```python
from build123d import *

# Parameters (mm, degrees)
F0_R     = 6.35
F0_R_2   = 3.175
F1_DEPTH = 2.3749
F2_R     = 0.2032
F3_R     = 0.2032
F4_R     = 0.2032
F5_R     = 0.2032


with BuildPart() as f1:
    # F0 (on Right) → F1 (new body, symmetric)
    with BuildSketch(Plane.YZ):
        Circle(F0_R)
        Circle(F0_R_2, mode=Mode.SUBTRACT)
    extrude(amount=F1_DEPTH, both=True)

    # F2
    f2_edges = [f1.edges().sort_by_distance(p)[0] for p in [
        (2.3749, -6.35, 0),
    ]]
    fillet(f2_edges, radius=F2_R)

    # F3
    f3_edges = [f1.edges().sort_by_distance(p)[0] for p in [
        (2.3749, -3.175, 0),
    ]]
    fillet(f3_edges, radius=F3_R)

    # F4
    f4_edges = [f1.edges().sort_by_distance(p)[0] for p in [
        (-2.3749, -6.35, 0),
    ]]
    fillet(f4_edges, radius=F4_R)

    # F5
    f5_edges = [f1.edges().sort_by_distance(p)[0] for p in [
        (-2.3749, -3.175, 0),
    ]]
    fillet(f5_edges, radius=F5_R)


solid = f1.part
```
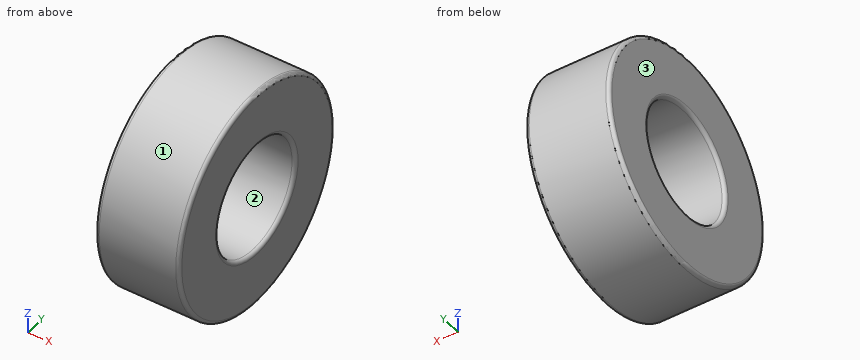
Part model, mm, in its own coordinate system. Face numbers are marked on the shaded views. Give positions to 0.01 mm unless a question says otherwise; leave off trailing zeros. Order: outer loops, then holes, each group sorted by start corner. A loop starts at its lowest first (then second) coordinate and runs counter-clockwise, first axis right, second up. Notation, with made-up numbers: (31, 44.5) - (55, 44.5) arc R30 ccw to (55, 68.5) - close; hole circle Ø4 at (15, 69.25). An arc over 180 degrees is marked (long way). Use one line per item in the form item = value.
Item 1: Slice it at C-C on x = 1.9. Give the cut face in (y, z) (3 decimals), and give its area (3 significant figures).
Solution:
outline = circle Ø12.7 at (0, 0); hole circle Ø6.35 at (0, 0)
area = 95.0 mm2
Item 2: Two-plate mould, pull along Z, no slides. Class the marked faces 1, 2 and 3: released by +Z, released by -Z, zero draft, split by the parting line, or undercut.
Solution:
face_1 = split by the parting line
face_2 = undercut
face_3 = zero draft
Item 3: Slice it at A-A on z = 0. Give the cut face in (x, y) (3 decimals).
Solution:
outline = (-2.375, -6.147) arc R0.203 ccw to (-2.172, -6.35) - (2.172, -6.35) arc R0.203 ccw to (2.375, -6.147) - (2.375, -3.378) arc R0.203 ccw to (2.172, -3.175) - (-2.172, -3.175) arc R0.203 ccw to (-2.375, -3.378) - close; (-2.375, 3.378) arc R0.203 ccw to (-2.172, 3.175) - (2.172, 3.175) arc R0.203 ccw to (2.375, 3.378) - (2.375, 6.147) arc R0.203 ccw to (2.172, 6.35) - (-2.172, 6.35) arc R0.203 ccw to (-2.375, 6.147) - close
Item 4: Pin check, flat tips, straight feed: pin 1 Ø1 at (x, y) = (1, -2) entering from +Z; pin 2 Ø3 at (y, z) = (-0.5, -1) entering from +X (3 decimals); pin 3 Ø1 at (x, y) = (1.5, -4) entering from -Z; pin 4 Ø1 at (x, y) = (1.5, -3.5) entering from +Z. Stop position of each tip, or through.
Solution:
pin_1 = 6.17
pin_2 = through
pin_3 = -5.3
pin_4 = 5.6
Item 5: Probe probe 1 along Z at (x, y) = (0, 0) (3 decimals); probe 2 along Y at (x, z) = (1.75, 2.25); probe 3 along Y at (x, z) = (-1, -1.5). List the from-to ranges inside material, lowest first. Write a range as from..to.
Solution:
probe_1 = -6.35..-3.175, 3.175..6.35
probe_2 = -5.94..-2.24, 2.24..5.94
probe_3 = -6.17..-2.8, 2.8..6.17
